```python
from build123d import *

# Parameters (mm, degrees)
ESQUISSE1_R                                = 19.45
ESQUISSE1_R_2                              = 16
BOSS_EXTRU_1_DEPTH                         = 3
ENL_V_MAT_EXTRU_1_DEPTH                    = 3
BOSS_EXTRU_2_DEPTH                         = 3
R_P_TITION_CIRCULAIRE1_COUNT               = 2
R_P_TITION_CIRCULAIRE1_ANGLE               = 120
R_P_TITION_CIRCULAIRE1_THE_OTHER_WAY_COUNT = 2
R_P_TITION_CIRCULAIRE1_THE_OTHER_WAY_ANGLE = 120
ESQUISSE2_R                                = 17.5
ENL_V_MAT_EXTRU_2_DEPTH                    = 0.5


with BuildPart() as part:
    # Esquisse1 → Boss.-Extru.1 (new body)
    with BuildSketch(Plane.XY):
        Circle(ESQUISSE1_R)
        Circle(ESQUISSE1_R_2, mode=Mode.SUBTRACT)
    extrude(amount=BOSS_EXTRU_1_DEPTH)

    # Esquisse1<12> → Enlèv. mat.-Extru.1 (cut)
    with BuildSketch(Plane.XY):
        with BuildLine():
            ThreePointArc((-1.498884406, 19.392159383), (-1.040009393, 18.369083508), (0, 17.95))
            Line((0, 17.95), (0, 19.45))
            ThreePointArc((0, 19.45), (-0.75, 19.435534467), (-1.498884406, 19.392159383))
        make_face()
        with BuildLine():
            Line((0, 19.45), (0, 17.95))
            ThreePointArc((0, 17.95), (1.040009393, 18.369083508), (1.498884406, 19.392159383))
            ThreePointArc((1.498884406, 19.392159383), (0.75, 19.435534467), (0, 19.45))
        make_face()
    enl_v_mat_extru_1 = extrude(amount=ENL_V_MAT_EXTRU_1_DEPTH, mode=Mode.SUBTRACT)

    # Esquisse1<13> → Boss.-Extru.2 (add)
    with BuildSketch(Plane.XY):
        with BuildLine():
            ThreePointArc((-1.498884406, 19.392159383), (-0.028925687, 20.949721076), (1.5, 19.45))
            ThreePointArc((1.5, 19.45), (1.499721076, 19.421074313), (1.498884406, 19.392159383))
            ThreePointArc((1.498884406, 19.392159383), (2.744536924, 19.255389299), (3.978796705, 19.038688946))
            ThreePointArc((3.978796705, 19.038688946), (3.994695659, 19.244071394), (4, 19.45))
            ThreePointArc((4, 19.45), (-0.205928606, 23.444695659), (-3.978796705, 19.038688946))
            ThreePointArc((-3.978796705, 19.038688946), (-2.744536924, 19.255389299), (-1.498884406, 19.392159383))
        make_face()
    boss_extru_2 = extrude(amount=BOSS_EXTRU_2_DEPTH)

    # Répétition circulaire1: Enlèv. mat.-Extru.1, Boss.-Extru.2 ×2 about axis
    r_p_tition_circulaire1_axis = Axis((0, 0, 3), (0, 0, -1))
    add([enl_v_mat_extru_1.rotate(r_p_tition_circulaire1_axis, i * R_P_TITION_CIRCULAIRE1_ANGLE / (R_P_TITION_CIRCULAIRE1_COUNT - 1)) for i in range(1, R_P_TITION_CIRCULAIRE1_COUNT)], mode=Mode.SUBTRACT)
    add([boss_extru_2.rotate(r_p_tition_circulaire1_axis, i * R_P_TITION_CIRCULAIRE1_ANGLE / (R_P_TITION_CIRCULAIRE1_COUNT - 1)) for i in range(1, R_P_TITION_CIRCULAIRE1_COUNT)])

    # Répétition circulaire1 the other way: Enlèv. mat.-Extru.1, Boss.-Extru.2 ×2 about axis
    r_p_tition_circulaire1_the_other_way_axis = Axis((0, 0, 3), (0, 0, 1))
    add([enl_v_mat_extru_1.rotate(r_p_tition_circulaire1_the_other_way_axis, i * R_P_TITION_CIRCULAIRE1_THE_OTHER_WAY_ANGLE / (R_P_TITION_CIRCULAIRE1_THE_OTHER_WAY_COUNT - 1)) for i in range(1, R_P_TITION_CIRCULAIRE1_THE_OTHER_WAY_COUNT)], mode=Mode.SUBTRACT)
    add([boss_extru_2.rotate(r_p_tition_circulaire1_the_other_way_axis, i * R_P_TITION_CIRCULAIRE1_THE_OTHER_WAY_ANGLE / (R_P_TITION_CIRCULAIRE1_THE_OTHER_WAY_COUNT - 1)) for i in range(1, R_P_TITION_CIRCULAIRE1_THE_OTHER_WAY_COUNT)])

    # Esquisse2 → Enlèv. mat.-Extru.2 (cut)
    with BuildSketch(Plane.XY.offset(3)):
        Circle(ESQUISSE2_R)
    extrude(amount=-ENL_V_MAT_EXTRU_2_DEPTH, mode=Mode.SUBTRACT)


solid = part.part
```
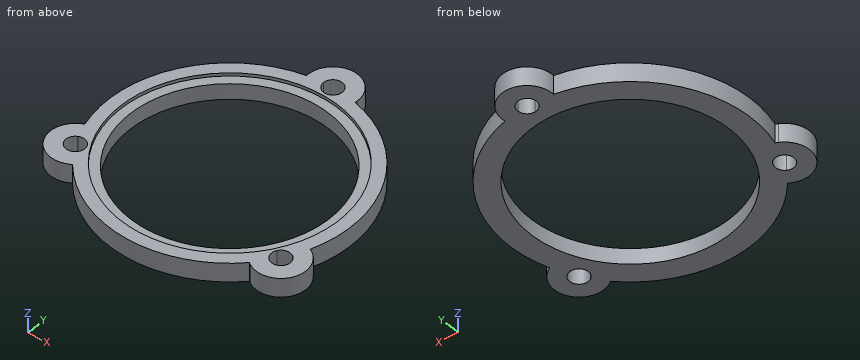
Input: part model. Units: mm. Frame: model coordinates. Coordinates: 2 decimals unless noted, no trailing zeros. Write each loop counter-clockwise with the first axis right and the second up, starting at its lowest first coordinate (ties: lowest second). Pieces come first, ordered by that corner, then holes.
1) Pin query (flat end, axial travel): pin 1 Ø10.5 at (x, y) = (-8, -0.5) entering from +Z. Return the tip coordinate at first contact, or that it passes through.
2) Section C-C on z = 0.75. Output: boundary loops of the cut face in (x, y) (3 decimals), and give its area (3 significant figures).
3) Material intervals for line 1 along Y through (x, z) = (0, 1.05); line 2 along Y through (x, z) = (0, 2.85); line 3 along X through (y, z) = (0, 0.5), sorted ascending.
4) Section B-B on x = 7. Output: boundary loops of the cut face in (y, z).
5) Section A-A on y = 0. Output: boundary loops of the cut face in (x, z), and give its area (3 significant figures).
Check result:
1. pin 1: passes through
2. outline: (-18.477, -6.074) arc R4 ccw (long way) to (-14.499, -12.965) arc R19.45 ccw to (14.499, -12.965) arc R4 ccw (long way) to (18.477, -6.074) arc R19.45 ccw to (3.979, 19.039) arc R4 ccw (long way) to (-3.979, 19.039) arc R19.45 ccw to start; hole (-17.594, -8.426) arc R1.5 ccw (long way) to (-17.544, -8.398) arc R1.5 ccw to start; hole circle Ø32 at (0, 0); hole (1.499, 19.392) arc R1.5 ccw to (1.5, 19.45) arc R1.5 ccw (long way) to start; hole (16.045, -10.994) arc R1.5 ccw to (16.094, -11.024) arc R1.5 ccw (long way) to start
2. area: 442 mm2
3. line 1: y = -19.45 to -16, 16 to 17.95, 20.95 to 23.45
3. line 2: y = -19.45 to -17.5, 17.5 to 17.95, 20.95 to 23.45
3. line 3: x = -19.45 to -16, 16 to 19.45
4. outline: (-18.15, 0) - (-14.39, 0) - (-14.39, 2.5) - (-16.04, 2.5) - (-16.04, 3) - (-18.15, 3) - close; (14.39, 0) - (18.15, 0) - (18.15, 3) - (16.04, 3) - (16.04, 2.5) - (14.39, 2.5) - close
5. outline: (-19.45, 0) - (-16, 0) - (-16, 2.5) - (-17.5, 2.5) - (-17.5, 3) - (-19.45, 3) - close; (16, 0) - (19.45, 0) - (19.45, 3) - (17.5, 3) - (17.5, 2.5) - (16, 2.5) - close
5. area: 19.2 mm2
